```python
from build123d import *

# Parameters (mm, degrees)
F0_R     = 9
F1_DEPTH = 15.1
F2_SIZE  = 2
F3_SIZE  = 1
F4_R     = 1.1
F5_DEPTH = 5
F6_R     = 2.5
F7_DEPTH = 11
F8_R     = 0.75
F9_DEPTH = 2


with BuildPart() as f1:
    # F0 (on Top) → F1 (new body)
    with BuildSketch(Plane.XY):
        Circle(F0_R)
    extrude(amount=F1_DEPTH)

    # F2
    f2_edges = [f1.edges().sort_by_distance(p)[0] for p in [
        (-9, 0, 15.1),
    ]]
    chamfer(f2_edges, length=F2_SIZE)

    # F3
    f3_edges = [f1.edges().sort_by_distance(p)[0] for p in [
        (-9, 0, 0),
    ]]
    chamfer(f3_edges, length=F3_SIZE)

    # F4 (on face) → F5 (cut)
    with BuildSketch(Plane(origin=(0, 0, 0), x_dir=(1, 0, 0), z_dir=(0, 0, -1))):
        with Locations((0, 6)):
            Circle(F4_R)
        with Locations((-6, 0)):
            Circle(F4_R)
        with Locations((0, -6)):
            Circle(F4_R)
        with Locations((6, 0)):
            Circle(F4_R)
    extrude(amount=-F5_DEPTH, mode=Mode.SUBTRACT)

    # F6 (on face) → F7 (join)
    with BuildSketch(Plane.XY.offset(15.1)):
        Circle(F6_R)
    extrude(amount=F7_DEPTH)

    # F8 (on face) → F9 (join)
    with BuildSketch(Plane(origin=(0, 0, 0), x_dir=(1, 0, 0), z_dir=(0, 0, -1))):
        Circle(F8_R)
    extrude(amount=F9_DEPTH)


solid = f1.part
```
Could you check a few things on this model? Use its own coordinates, in mm. A direction names the side the tool comes from. Give positions to 0.01 mm unless a question says otherwise; leave off trailing zeros. Write each loop counter-clockwise with the first axis right and the second up, starting at its lowest first coordinate (ties: lowest second). Pieces come first, ordered by that corner, then holes. Notation, with made-up numbers: (0, -32.75) -> (24, -32.75) arc R18 cw to (24, -14.75) -> close; hole circle Ø1 at (-22.5, -26). An arc over 180 degrees is marked (long way). Write each question's results on one line, items separated by ' | '.
1. Will these pins go through, and if not, where does the flat tip stop? pin 1 Ø8 at (x, y) = (4.5, -5) entering from +Z; pin 2 Ø1.5 at (x, y) = (-5, 7) entering from +Z; pin 3 Ø1.1 at (x, y) = (0, -6) entering from -Z.
Check sheet entries:
pin 1: stops at z = 15.1 | pin 2: stops at z = 14.25 | pin 3: stops at z = 5
2. I want a section at A-A, the plane x = 0. Write out the boundary of the cut face in (y, z).
Check sheet entries:
outline: (-9, 1) -> (-8, 0) -> (-7.1, 0) -> (-7.1, 5) -> (-4.9, 5) -> (-4.9, 0) -> (-0.75, 0) -> (-0.75, -2) -> (0.75, -2) -> (0.75, 0) -> (4.9, 0) -> (4.9, 5) -> (7.1, 5) -> (7.1, 0) -> (8, 0) -> (9, 1) -> (9, 13.1) -> (7, 15.1) -> (2.5, 15.1) -> (2.5, 26.1) -> (-2.5, 26.1) -> (-2.5, 15.1) -> (-7, 15.1) -> (-9, 13.1) -> close
3. I want a section at B-B, the plane z = 18.25. Write out the boundary of the cut face in (x, y).
Check sheet entries:
outline: circle Ø5 at (0, 0)
4. I need wall thicknesses on L1, parallel to Y at x = 0, z = 2.45; L2, parallel to Y at x = 0.75, z = 4; L3, parallel to Z at x = 4.5, y = 1.25. Which ranges of each line are inside material? Lowest first, please.
Check sheet entries:
L1: y = -9 to -7.1, -4.9 to 4.9, 7.1 to 9 | L2: y = -8.97 to -6.8, -5.2 to 5.2, 6.8 to 8.97 | L3: z = 0 to 15.1
5. If we mould it in two halves opening along Y, with no side actions, what happens to faces 1 (the cylindrical face through (-1.172, 8.923, 6.965)), 2 (the cylindrical face through (7.016, 0.421, 2.465)), 3 (the flat face through (0, 0, -2))? For each: released by +Y, released by -Y, zero draft, split by the parting line, or undercut.
Check sheet entries:
face 1: split by the parting line | face 2: undercut | face 3: zero draft
6. On a 3-axis mill with a long thin cutter (end or side, diameter ignored), from which of +Z, -Z, +X, -X, +Y, -Y can I reach the whole of each face in a straight line? I mean faces 4 (the cylindrical face through (-0.75, -0.03, -0.99)), 5 (the flat face through (0, -3, 15.1)), 6 (the flat face through (0, 0, 26.1)). Say none if no direction works.
Check sheet entries:
face 4: -Z | face 5: +Z | face 6: +Z, +X, -X, +Y, -Y
7. I want a section at C-C, the plane z = 9. Write out the boundary of the cut face in (x, y).
Check sheet entries:
outline: circle Ø18 at (0, 0)
